Here's how the part is built. I have some questions about the finished solid (model axes, mm). A direction names the side the tool comes from. Coordinates: 2 decimals unless noted, no trailing zeros.
(1) Imagine slicing it at A-A, the plane x = -76.2. State how many separate pieces and enclosed holes the cut face has, plus the area to 3 significant figures.
(2) Please list where these lines run through material, in increasing order: probe 1 along Y at (x, z) = (76, 18); probe 2 along X at (y, z) = (-31.75, 1.5); probe 3 along Y at (x, z) = (-6, 15) (3 decimals).
(3) For pin 1 Ø5 at (x, y) = (9, -16) entering from +Z; pin 2 Ø11 at (x, y) = (0, -31.75) entering from +Z; pin 3 Ø8 at (y, z) = (-3.5, 19) entering from -X (3 decimals); pin 4 Ø7.5 at (x, y) = (-76.2, -31.75) entering from -Z, each with a flat end and sliding along its axis, tell me the tip position at first contact or that it passes through.
(4) Thinking about a two-plate mould opening in Y: for faces 1 (the flat face through (20, -44.45, 12)), 2 (the cylindrical face through (58.876, 14.347, 13.279)), 3 (the flat face through (20, 44.45, 12)), which applies, released by +Y, released by -Y, zero draft, split by the parting line, or undercut?
(5) Which directions (+Z, -Z, +X, -X, +Y, -Y) give clear straight access to the entire face, cutting with the end or side of a thin tool? Please do faces 4 (the flat face through (-1, 20, 0)), 5 (the flat face through (-60.325, 0, 4)).
```python
from build123d import *

# Parameters (mm, degrees)
F0_W     = 190.5
F0_H     = 88.9
F0_R     = 4.7625
F0_W_2   = 120.65
F0_H_2   = 31.75
F1_DEPTH = 50.8
F3_DEPTH = 88.901
F5_R     = 2895.6
F4_R     = 2895.6
F7_R     = 5.08


with BuildPart() as f1:
    # F0 (on Top) → F1 (new body)
    with BuildSketch(Plane.XY):
        Rectangle(F0_W, F0_H)
        with Locations((-76.2, -31.75)):
            Circle(F0_R, mode=Mode.SUBTRACT)
        with Locations((0, -31.75)):
            Circle(F0_R, mode=Mode.SUBTRACT)
        with Locations((76.2, -31.75)):
            Circle(F0_R, mode=Mode.SUBTRACT)
        with Locations((-76.2, 31.75)):
            Circle(F0_R, mode=Mode.SUBTRACT)
        Rectangle(F0_W_2, F0_H_2, mode=Mode.SUBTRACT)
        with Locations((0, 31.75)):
            Circle(F0_R, mode=Mode.SUBTRACT)
        with Locations((76.2, 31.75)):
            Circle(F0_R, mode=Mode.SUBTRACT)
    extrude(amount=F1_DEPTH)

    # F2 (on face) → F3 (cut, through all)
    with BuildSketch(Plane.XZ.offset(44.45)):
        Polygon((-129.30572, 83.835296), (-95.25, 3.175), (95.25, 31.75), (118.781321, 86.451776), align=None)
    extrude(amount=-F3_DEPTH, mode=Mode.SUBTRACT)

    # F5 (on face) → F6 section 0
    with BuildSketch(Plane(origin=(-95.25, 0, 0), x_dir=(0, -1, 0), z_dir=(-1, 0, 0))):
        with Locations((0, 2898.433807)):
            Circle(F5_R)
    # F4 (on face) → F6 section 1
    with BuildSketch(Plane.YZ.offset(95.25)):
        with Locations((0, 2927.008807)):
            Circle(F4_R)
    loft(mode=Mode.SUBTRACT)

    # F7
    f7_edges = [f1.edges().sort_by_distance(p)[0] for p in [
        (60.325, 15.875, 13.106787),
        (60.325, -15.875, 13.106787),
        (-60.325, -15.875, 4.058037),
        (-60.325, 15.875, 4.058037),
    ]]
    fillet(f7_edges, radius=F7_R)


solid = f1.part
```
Recorded:
1. separate pieces: 3
1. enclosed holes: 0
1. area: 404 mm2
2. probe 1: y = -44.45 to -36.51, -26.99 to 26.99, 36.51 to 44.45
2. probe 2: x = -95.25 to -80.96, -71.44 to -4.76, 4.76 to 71.44, 80.96 to 95.25
2. probe 3: y = -44.45 to -15.875, 15.875 to 44.45
3. pin 1: stops at z = 18.89
3. pin 2: stops at z = 18.12
3. pin 3: stops at x = 60.325
3. pin 4: passes through
4. face 1: released by -Y
4. face 2: undercut
4. face 3: released by +Y
5. face 4: -Z, +X, -X, +Y, -Y
5. face 5: +Z, -Z
